Job drawing, mm, ordinate dimensions from the low corner. One solid piece. A direction names the side the tool comes from. Coordinates: 2 decimals unless noted, no trailing zeros. Loops run counter-clockwise (first coordinate to the right, second up) from the corner with the lowest first, then second, coordinate; pieces in that order, holes last. Notation, with made-up numbers: (-27, 24) -> (-2, 24) arc R27 ccw to (-2, 62) -> close; hole circle Ø6 at (-23.75, 61). An arc over 180 degrees is marked (long way). Answer as CSV lines item,"result". Start each with the question number.
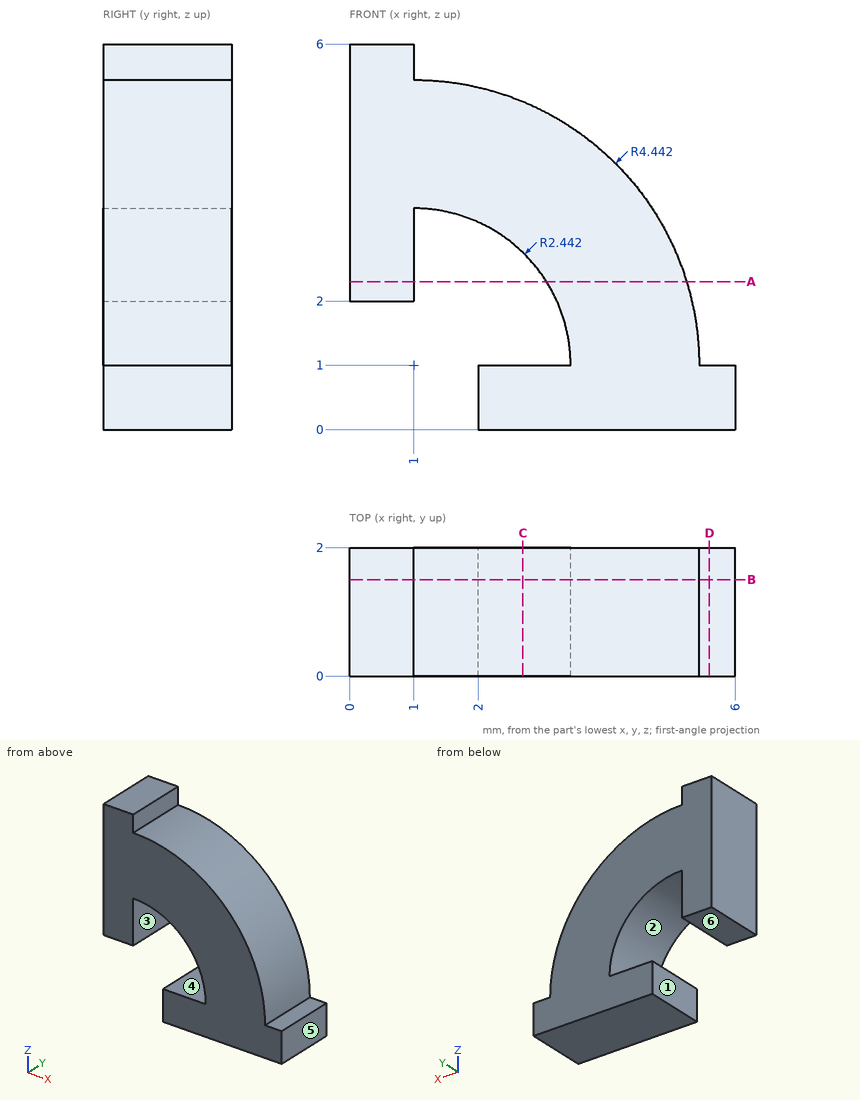
Item 1: Wall check: probe 1 along Z at (x, y) = (5.75, 0.7); probe 2 along X at (y, z) = (0.8, 2.3); probe 3 along X at (y, z) = (0.25, 0.8). Give the ranges that are in metal, low to high.
Item 2: Saw through at C-C (x = 2.7). Write the cut outline in (y, z).
Item 3: Saw through at D-D (x = 5.6). Write the cut outline in (y, z).
Item 4: Two-plate mould, pull along Z, no slides. Class the marked faces 4, 5 and 6: pulls with the +Z half, pulls with the -Z half, needs draft (parallel to the pull), parting line crosses it, or undercut.
Item 5: Saw through at A-A (z = 2.3). Write the cut outline in (x, y).
Item 6: Which spindle directions (+Z, -Z, +X, -X, +Y, -Y) get a long thin tool onto all of the face, cutting with end or side? Do the marked faces 1, 2 and 3. Say none if no direction does.
Item 7: Saw through at B-B (y = 1.5). Write the cut outline in (x, z).
Item 8: Flat gauge pins, fed straight in: pin 1 Ø0.5 at (y, z) = (1.5, 0.5) entering from -X; pin 2 Ø0.8 at (x, y) = (0.5, 1.5) entering from -Z. Where does each tip first touch, or does it go through?
Geometry check:
1,probe 1,"0 to 1"
1,probe 2,"0 to 1, 3.07 to 5.25"
1,probe 3,"2 to 6"
2,outline,"(0, 0) -> (2, 0) -> (2, 1) -> (0, 1) -> close; (0, 2.75) -> (2, 2.75) -> (2, 5.1) -> (0, 5.1) -> close"
3,outline,"(0, 0) -> (2, 0) -> (2, 1) -> (0, 1) -> close"
4,face 4,"undercut"
4,face 5,"needs draft"
4,face 6,"pulls with the -Z half"
5,outline,"(0, 0) -> (1, 0) -> (1, 2) -> (0, 2) -> close; (3.07, 0) -> (5.25, 0) -> (5.25, 2) -> (3.07, 2) -> close"
6,face 1,"-Z, -X, +Y, -Y"
6,face 2,"+Y, -Y"
6,face 3,"-Z, +Y, -Y"
7,outline,"(0, 2) -> (1, 2) -> (1, 3.44) arc R2.44 cw to (3.44, 1) -> (2, 1) -> (2, 0) -> (6, 0) -> (6, 1) -> (5.44, 1) arc R4.44 ccw to (1, 5.44) -> (1, 6) -> (0, 6) -> close"
8,pin 1,"x = 2"
8,pin 2,"z = 2"
